Check sheet for the drawn part. Datum: minimum x, y, z corner. Units: mm. A direction names the side the tool comes from. Give positions to 0.01 mm unless a question says otherwise; leave off trailing zeros. Order: outer loops, then holes, each group sorted by start corner. A loop starts at its lowest first (then second) coordinate and runs counter-clockwise, first axis right, second up. Notation, with made-up numbers: M -13,-25 L 43,-25 A13 cw 43,-17 Z; hole C 52,23.25 d5. An arc over 180 degrees is marked long. Put each result on its own line as item: value. Start each with the question number.
Q1. Material ranges on L1, parallel to Z at x = 10, y = 10.5; L2, parallel to X at y = 57.5, z = 25.5; L3, parallel to Y at x = 18.25, z = 9.5, recorded low to high.
Q2. Section check A-A on y = 12.5. Record the cut outline in (x, z), then the cut area to 3 significant figures.
Q3. Section check D-D on y = 76.5. Record the cut outline in (x, z).
Q4. Go/stop test with flat-tipped pins: pin 1 (5 mm diameter, centred on x = 4.5, z = 30.5, fed in from +Y); pin 2 (11 mm diameter, centred on x = 14, y = 30, fed in from -Z); pin 3 (5 mm diameter, centred on x = 18, z = 6.5, fed in from -Y). Record where each tip stops, or that it passes through.
Q5. Access from +Z, -Z, +X, -X, +Y, -Y to the whole of each face (thin tool, end or side, straight path). Record for the marked faces 1, 2 and 3.
Q6. Section check B-B on z = 29. Record the cut outline in (x, y).
Q7. Section check C-C on x = 17.5. Record the cut outline in (y, z), then the cut area to 3 significant figures.
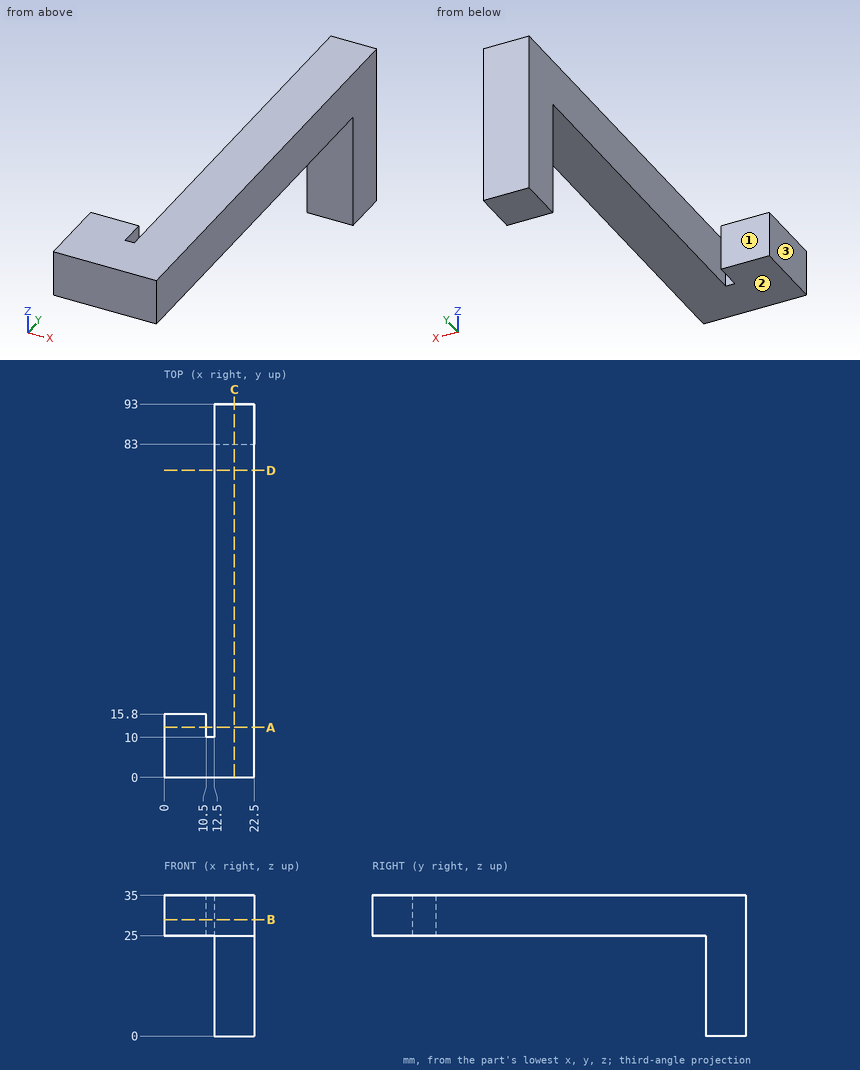
Results found:
1. L1: z = 25 to 35
1. L2: x = 12.5 to 22.5
1. L3: y = 83 to 93
2. outline: M 0,25 L 10.5,25 L 10.5,35 L 0,35 Z; M 12.5,25 L 22.5,25 L 22.5,35 L 12.5,35 Z
2. area: 205 mm^2
3. outline: M 12.5,25 L 22.5,25 L 22.5,35 L 12.5,35 Z
4. pin 1: stops at y = 15.8
4. pin 2: stops at z = 25
4. pin 3: stops at y = 83
5. face 1: +Z, -Z, -X, +Y
5. face 2: -Z, +X, -X, -Y
5. face 3: +Z, -Z, -X, +Y, -Y
6. outline: M 0,0 L 22.5,0 L 22.5,93 L 12.5,93 L 12.5,10 L 10.5,10 L 10.5,15.8 L 0,15.8 Z
7. outline: M 0,25 L 83,25 L 83,0 L 93,0 L 93,35 L 0,35 Z
7. area: 1,180 mm^2
